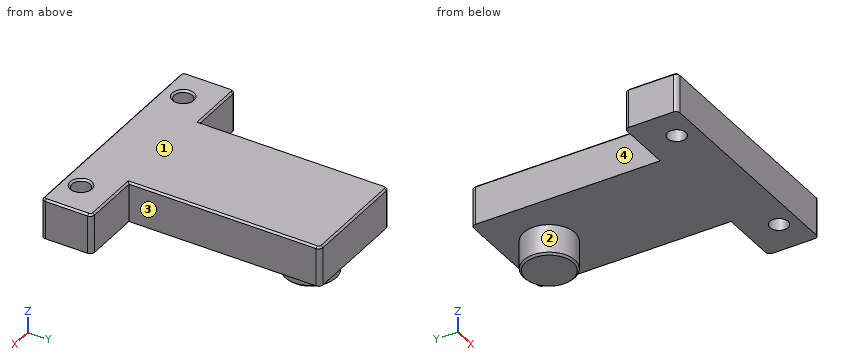
from build123d import *

# Parameters (mm, degrees)
EXTRUDE_1_DEPTH     = 2.2
FILLET_1_R          = 0.23
SKETCH_4_R          = 1.41
EXTRUDE_2_DEPTH     = 1.65
CHAMFER_1_SIZE      = 0.1
SKETCH_5_R          = 0.5
CUT_EXTRUDE_1_DEPTH = 2.2
CHAMFER_2_SIZE      = 0.1


with BuildPart() as part:
    # 草图2 → 凸台-拉伸1 (new body)
    with BuildSketch(Plane.XY):
        Polygon((73.787, 72.009), (76.962, 72.009), (76.962, 82.423), (83.058, 82.423), (83.058, 71.882), (86.36, 71.882), (86.36, 69.088), (82.804, 69.088), (77.343, 69.088), (73.787, 69.088), align=None)
    extrude(amount=EXTRUDE_1_DEPTH)

    # 圆角1
    fillet_1_edges = [part.edges().sort_by_distance(p)[0] for p in [
        (73.787, 72.009, 1.1),
        (76.962, 82.423, 1.1),
        (83.058, 82.423, 1.1),
        (86.36, 71.882, 1.1),
        (86.36, 69.088, 1.1),
        (73.787, 69.088, 1.1),
    ]]
    fillet(fillet_1_edges, radius=FILLET_1_R)

    # 草图4 → 凸台-拉伸2 (add)
    with BuildSketch(Plane.XY):
        with Locations(Location((80.00000002, 80.00000002, 0), (0, 0, 180))):
            Circle(SKETCH_4_R)
    extrude(amount=-EXTRUDE_2_DEPTH)

    # 倒角1
    chamfer_1_edges = [part.edges().sort_by_distance(p)[0] for p in [
        (83.058, 77.0375, 2.2),
        (80.0735, 69.088, 2.2),
        (73.787, 70.5485, 2.2),
        (75.4895, 72.009, 2.2),
        (86.36, 70.485, 2.2),
        (84.594, 71.882, 2.2),
        (80.01, 82.423, 2.2),
        (76.962, 77.101, 2.2),
        (86.29263456, 71.81463456, 2.2),
        (86.29263456, 69.15536544, 2.2),
        (82.99063456, 82.35563456, 2.2),
        (77.02936544, 82.35563456, 2.2),
        (73.85436544, 71.94163456, 2.2),
        (73.85436544, 69.15536544, 2.2),
        (81.41000002, 80.00000002, -1.65),
    ]]
    chamfer(chamfer_1_edges, length=CHAMFER_1_SIZE)

    # 草图5 → 切除-拉伸1 (cut)
    with BuildSketch(Plane.XY):
        with Locations(Location((75.565, 70.231, 0), (0, 0, 180))):
            Circle(SKETCH_5_R)
        with Locations(Location((84.455, 70.104, 0), (0, 0, 180))):
            Circle(SKETCH_5_R)
    extrude(amount=CUT_EXTRUDE_1_DEPTH, mode=Mode.SUBTRACT)

    # 倒角2
    chamfer_2_edges = [part.edges().sort_by_distance(p)[0] for p in [
        (76.065, 70.231, 2.2),
        (84.955, 70.104, 2.2),
    ]]
    chamfer(chamfer_2_edges, length=CHAMFER_2_SIZE)


solid = part.part
Read the model definition and answer for the solid it produces. Units are mm, in the model's axes. Face numbers are marked on the shaded views. A direction names the side the tool comes from. Give positions to 0.01 mm unless a question says otherwise; leave off trailing zeros. Loops run counter-clockwise (first coordinate to the right, second up) from the corner with the lowest first, then second, coordinate; pieces in that order, holes last. Notation, with made-up numbers: (-17.5, 32.5) - (30.5, 32.5) arc R21 ccw to (30.5, 39.5) - close; hole circle Ø1 at (36, -4.75). An arc over 180 degrees is marked (long way). Answer as CSV lines item,"result". Start each with the question number.
1) Straight lines are drawn through the part: L1, parallel to X at y = 70, z = 1.6; L2, parallel to X at y = 70.5, z = 1.35; L3, parallel to X at y = 75.75, z = 1.9. For each, find the intervals that lie inside material, in ascending order. Write a range as from..to.
2) Find section C-C (z = 0.75). Write down the section's boundary in (x, y) (3 decimals), then the cut area to 3 significant figures.
3) Find section B-B (x = 80). Write down the section's boundary in (y, z), then the cut area to 3 significant figures.
4) Find section A-A (y = 80). Write down the section's boundary in (x, z).
5) Which of the six approach directions +Z, -Z, +X, -X, +Y, -Y give full straight-line access (tool end or side, diameter ignored) to the marked faces 1, 2, 3 and 4?
6) Find section D-D (z = -0.9). Write down the section's boundary in (x, y).
7) Each of these flat-tipped pins is pushed along its axis until it touches: pin 1 Ø1.5 at (x, y) = (76.5, 74) entering from -Z; pin 2 Ø1.7 at (x, z) = (76, 0.5) entering from +Y; pin 3 Ø0.6 at (y, z) = (79, 1) entering from -X. Where does it stop, or does it pass through?
Findings below:
1,L1,"73.79..75.12, 76.01..83.97, 84.94..86.36"
1,L2,"73.79..75.14, 75.99..84.15, 84.76..86.36"
1,L3,"76.96..83.06"
2,outline,"(73.787, 69.318) arc R0.23 ccw to (74.017, 69.088) - (86.13, 69.088) arc R0.23 ccw to (86.36, 69.318) - (86.36, 71.652) arc R0.23 ccw to (86.13, 71.882) - (83.058, 71.882) - (83.058, 82.193) arc R0.23 ccw to (82.828, 82.423) - (77.192, 82.423) arc R0.23 ccw to (76.962, 82.193) - (76.962, 72.009) - (74.017, 72.009) arc R0.23 ccw to (73.787, 71.779) - close; hole circle Ø1 at (75.565, 70.231); hole circle Ø1 at (84.455, 70.104)"
2,area,"98.2 mm^2"
3,outline,"(69.09, 0) - (78.59, 0) - (78.59, -1.55) - (78.69, -1.65) - (81.31, -1.65) - (81.41, -1.55) - (81.41, 0) - (82.42, 0) - (82.42, 2.1) - (82.32, 2.2) - (69.19, 2.2) - (69.09, 2.1) - close"
3,area,"34.0 mm^2"
4,outline,"(76.96, 0) - (78.59, 0) - (78.59, -1.55) - (78.69, -1.65) - (81.31, -1.65) - (81.41, -1.55) - (81.41, 0) - (83.06, 0) - (83.06, 2.1) - (82.96, 2.2) - (77.06, 2.2) - (76.96, 2.1) - close"
5,face 1,"+Z, +X, -X, +Y, -Y"
5,face 2,"-Z"
5,face 3,"+Z, -Z, +X, +Y"
5,face 4,"+Z, -Z, -X, +Y"
6,outline,"circle Ø2.82 at (80, 80)"
7,pin 1,"z = 0"
7,pin 2,"y = 72.01"
7,pin 3,"x = 76.96"
